Answer from the drawing. Dimensions are ordinates in mm from the lowest x, y and z of the part. Round coordinates to 2 decimals unless told otherwise and drop trailing zeros. Order: outer loops, then holes, each group sorted by start corner. A loop starts at its lowest first (then second) coordinate and runs counter-clockwise, first axis right, second up. Notation, with made-up numbers: (87, -10.75) - (125, -10.75) arc R17 ccw to (125, -2.75) - close; hole circle Ø2 at (33, 82.25). An arc over 180 degrees is marked (long way). One line per question, with ' | ' between items. Start each with the question number.
1) Straight lines are drawn through the part: line 1 (X direction, y = 71, z = 1.8); line 2 (Y direction, x = 211, z = 4.7); line 3 (X direction, y = 38.5, z = 1.65). For each, find the intervals that lie inside material, in ascending order. Write a range as from..to.
2) The part is cut by section C-C, the plane x = 201.5. Give the vertices of the cut face in (y, z), plus the area to 3 significant figures.
3) The part is cut by section A-A, the plane z = 1.3. Give the vertices of the cut face in (x, y).
4) Flat-ended cylindrical pins translate along their axes: pin 1 (2.5 mm diameter, centred on x = 197, z = 2.5, fed in from -Y); pin 2 (1.6 mm diameter, centred on y = 33.5, z = 2.5, fed in from +X). Find the tip coordinate at first contact, or state that the pin passes through.
5) The part is cut by section B-B, the plane y = 36.5. Give the vertices of the cut face in (x, z).
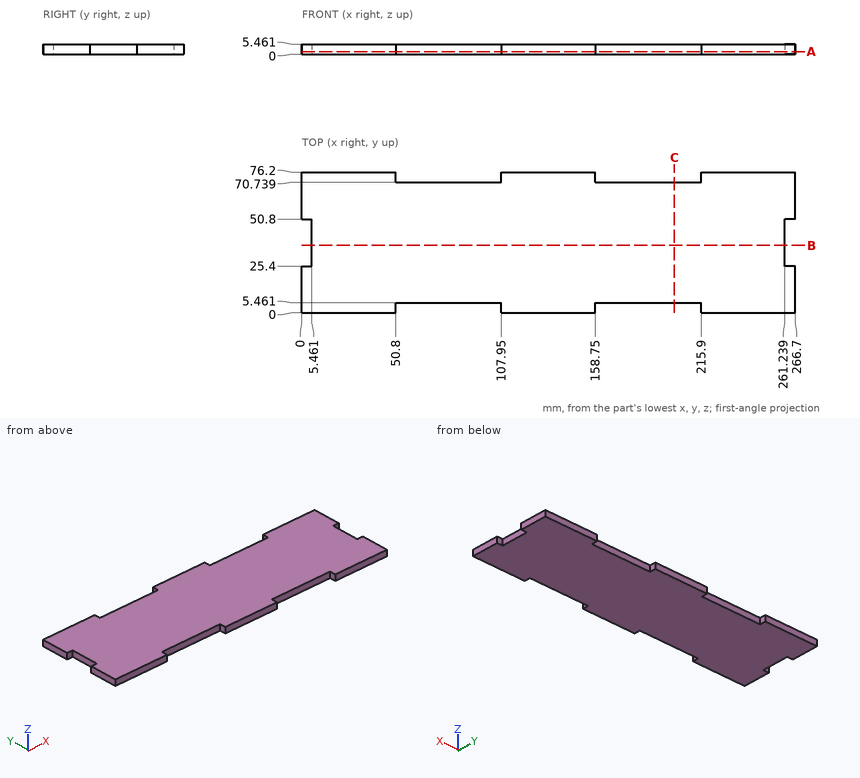
Values:
1) line 1: x = 0..50.8, 107.95..158.75, 215.9..266.7 | line 2: y = 5.46..70.74 | line 3: x = 5.46..261.24
2) outline: (5.46, 0) - (70.74, 0) - (70.74, 5.46) - (5.46, 5.46) - close | area: 356 mm^2
3) outline: (0, 0) - (50.8, 0) - (50.8, 5.46) - (107.95, 5.46) - (107.95, 0) - (158.75, 0) - (158.75, 5.46) - (215.9, 5.46) - (215.9, 0) - (266.7, 0) - (266.7, 25.4) - (261.24, 25.4) - (261.24, 50.8) - (266.7, 50.8) - (266.7, 76.2) - (215.9, 76.2) - (215.9, 70.74) - (158.75, 70.74) - (158.75, 76.2) - (107.95, 76.2) - (107.95, 70.74) - (50.8, 70.74) - (50.8, 76.2) - (0, 76.2) - (0, 50.8) - (5.46, 50.8) - (5.46, 25.4) - (0, 25.4) - close
4) pin 1: stops at y = 5.46 | pin 2: stops at x = 261.24
5) outline: (5.46, 0) - (261.24, 0) - (261.24, 5.46) - (5.46, 5.46) - close
